Autodesk Inventor part; units mm, degrees
ref_plane "YZ Plane" through (0, 0, 0) normal (1, 0, 0) x (0, 1, 0)
ref_plane "XZ Plane" through (0, 0, 0) normal (0, 1, 0) x (-1, 0, 0)
ref_plane "XY Plane" through (0, 0, 0) normal (0, 0, 1) x (1, 0, 0)
sketch "Sketch1" plane through (0, 0, 0) normal (0, 1, 0) x (-1, 0, 0)
  line L0 (3.1278, 4.0625) -> (3.1278, -5.9375)
  line L1 (3.1278, -5.9375) -> (-22.8722, -5.9375)
  line L2 (-22.8722, -5.9375) -> (-22.8722, 4.0625)
  line L3 (-22.8722, 4.0625) -> (3.1278, 4.0625)
  circle A0 centre (-3.3722, -0.9375) radius 1.9
  line L4 (-9.8722, -5.9375) -> (-9.8722, 8.6537)
  circle A1 centre (-16.3722, -0.9375) radius 1.9
  point P0 (0, 0)
  dimension "d0" = 10
  dimension "d1" = 26
  dimension "d2" = 3.8
  dimension "d4" = 6.5
  dimension "d5" = 6.5
  dimension "d6" = 13
extrude "Extrusion1" add sketch "Sketch1" along normal blind 3.5
properties part number "prepoj"
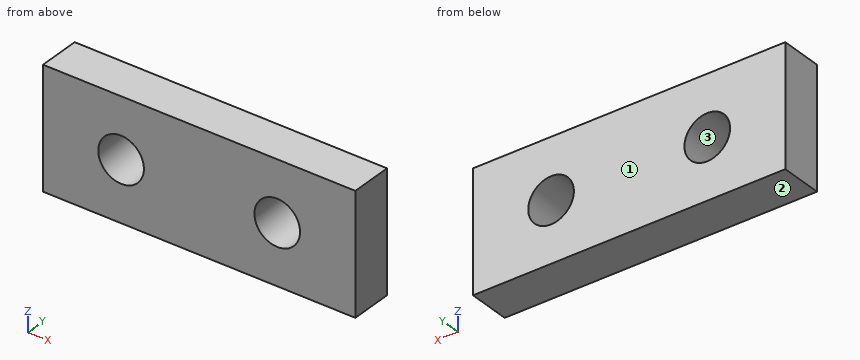
Can you work these out from the model? Positions are in its coordinate system, mm. Face numbers are marked on the shaded views. Round coordinates to 2 decimals unless told otherwise and drop trailing zeros. Loops run counter-clockwise (first coordinate to the right, second up) from the corner with the lowest first, then second, coordinate; pieces in that order, holes last.
Item 1: Please list where these lines run through material, in increasing order: L1, parallel to X at y = 0.75, z = 0; L2, parallel to X at y = 2.5, z = -2; L3, parallel to Z at x = 3.25, y = 0.45.
Item 2: Suppose I cut it at B-B, the plane x = 2.75. Write out the boundary of the cut face in (y, z).
Item 3: Suppose I cut it at C-C, the plane y = 0.8. Write out the boundary of the cut face in (x, z).
Item 4: Suppose I cut it at A-A, the plane z = -1.25. Write out the boundary of the cut face in (x, y).
Item 5: Suppose I cut it at D-D, the plane x = 17.75. Write out the boundary of the cut face in (y, z), then the cut area to 3 significant figures.
Item 6: If we mould it in two halves opening along Z, with no side actions, what happens to the marked faces 1, 2 and 3? For each: +Z half, -Z half, draft (parallel to the pull), parting line (faces both ways), or undercut.
Reported:
1. L1: x = -3.13 to 1.72, 5.02 to 14.72, 18.02 to 22.87
1. L2: x = -3.13 to 1.8, 4.95 to 14.8, 17.95 to 22.87
1. L3: z = -5.94 to -2.83, 0.96 to 4.06
2. outline: (0, -5.94) - (3.5, -5.94) - (3.5, -2.73) - (0, -2.73) - close; (0, 0.86) - (3.5, 0.86) - (3.5, 4.06) - (0, 4.06) - close
3. outline: (-3.13, -5.94) - (22.87, -5.94) - (22.87, 4.06) - (-3.13, 4.06) - close; hole circle Ø3.8 at (3.37, -0.94); hole circle Ø3.8 at (16.37, -0.94)
4. outline: (-3.13, 0) - (1.5, 0) - (1.5, 3.5) - (-3.13, 3.5) - close; (5.25, 0) - (14.5, 0) - (14.5, 3.5) - (5.25, 3.5) - close; (18.25, 0) - (22.87, 0) - (22.87, 3.5) - (18.25, 3.5) - close
5. outline: (0, -5.94) - (3.5, -5.94) - (3.5, -2.25) - (0, -2.25) - close; (0, 0.37) - (3.5, 0.37) - (3.5, 4.06) - (0, 4.06) - close
5. area: 25.8 mm2
6. face 1: draft
6. face 2: -Z half
6. face 3: undercut
